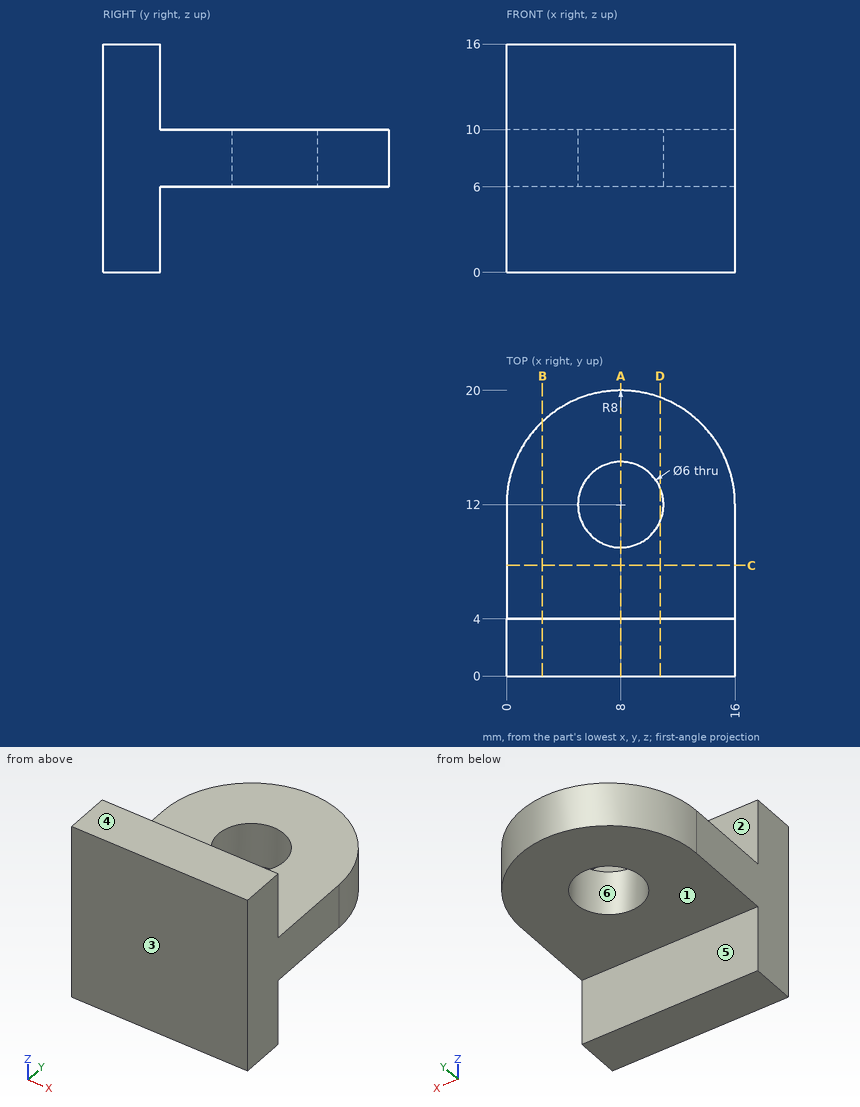
Geometry check sheet. Reference: drawing and pictorial views, mm from the part's lowest x, y, z. A direction names the side the tool comes from. Give positions to 0.01 mm unless a question says otherwise; leave off trailing zeros. Loops run counter-clockwise (first coordinate to the right, second up) from the corner with the lowest first, then second, coordinate; pieces in that order, holes last.
1. Mould release check, pull along Y, two halves, no side actions. Record for the marked faces 4, 5 and 6: released by +Y, released by -Y, zero draft, split by the parting line, or undercut.
2. Section check C-C, the plane y = 7.75. Enter the section's corners in (x, z), then the cut area to 3 significant figures.
3. Go/stop test with flat-tipped pins: pin 1 Ø5 at (x, y) = (7.5, 10.5) entering from +Z; pin 2 Ø8 at (x, y) = (4.5, 12) entering from -Z; pin 3 Ø5 at (y, z) = (13, 13) entering from +X; pin 4 Ø3 at (x, z) = (7, 2) entering from +Y. Record where each tip stops, or that it passes through.
4. Thickness scan on line 1 (Y direction, x = 8, z = 9.1); line 2 (Y direction, x = 2, z = 11.5); line 3 (Z direction, x = 9.25, y = 17). Record the ranges inside material, lowest first.
5. Section check B-B, the plane x = 2.5. Enter the section's corners in (y, z).
6. Section check D-D, the plane x = 10.75. Enter the section's corners in (y, z).
7. Set-up check for the marked faces 1, 2 and 3: record each of +Z, -Z, +X, -X, +Y, -Y from which the full face is reachable in a straight line by a thin tool's end or side.
8. Section check A-A, the plane x = 8. Enter the section's corners in (y, z), then the cut area to 3 significant figures.
Geometry says:
1. face 4: zero draft
1. face 5: released by +Y
1. face 6: undercut
2. outline: (0, 6) - (16, 6) - (16, 10) - (0, 10) - close
2. area: 64.0 mm2
3. pin 1: stops at z = 10
3. pin 2: stops at z = 6
3. pin 3: passes through
3. pin 4: stops at y = 4
4. line 1: y = 0 to 9, 15 to 20
4. line 2: y = 0 to 4
4. line 3: z = 6 to 10
5. outline: (0, 0) - (4, 0) - (4, 6) - (17.81, 6) - (17.81, 10) - (4, 10) - (4, 16) - (0, 16) - close
6. outline: (0, 0) - (4, 0) - (4, 6) - (10.8, 6) - (10.8, 10) - (4, 10) - (4, 16) - (0, 16) - close; (13.2, 6) - (19.51, 6) - (19.51, 10) - (13.2, 10) - close
7. face 1: -Z, +X, -X, +Y
7. face 2: +Z, +X, -X, +Y
7. face 3: +Z, -Z, +X, -X, -Y
8. outline: (0, 0) - (4, 0) - (4, 6) - (9, 6) - (9, 10) - (4, 10) - (4, 16) - (0, 16) - close; (15, 6) - (20, 6) - (20, 10) - (15, 10) - close
8. area: 104 mm2
